from build123d import *

# Parameters (mm, degrees)
SKETCH1_W           = 75
SKETCH1_H           = 45
SKETCH1_R           = 14
SKETCH1_R_2         = 1.6
BOSS_EXTRUDE1_DEPTH = 3
FILLET2_R           = 5
SKETCH2_R           = 1.6
CUT_EXTRUDE1_DEPTH  = 44.834917589


with BuildPart() as part:
    # Sketch1 → Boss-Extrude1 (new body)
    with BuildSketch(Plane.XY):
        Rectangle(SKETCH1_W, SKETCH1_H)
        Circle(SKETCH1_R, mode=Mode.SUBTRACT)
        with Locations((-15.5, 15.5)):
            Circle(SKETCH1_R_2, mode=Mode.SUBTRACT)
        with Locations((15.5, 15.5)):
            Circle(SKETCH1_R_2, mode=Mode.SUBTRACT)
        with Locations((15.5, -15.5)):
            Circle(SKETCH1_R_2, mode=Mode.SUBTRACT)
        with Locations((-15.5, -15.5)):
            Circle(SKETCH1_R_2, mode=Mode.SUBTRACT)
    extrude(amount=BOSS_EXTRUDE1_DEPTH)

    # Fillet2
    fillet2_edges = [part.edges().sort_by_distance(p)[0] for p in [
        (37.5, -22.5, 1.5),
        (-37.5, -22.5, 1.5),
        (-37.5, 22.5, 1.5),
        (37.5, 22.5, 1.5),
    ]]
    fillet(fillet2_edges, radius=FILLET2_R)

    # Sketch2 → Cut-Extrude1 (cut, through all)
    with BuildSketch(Plane.XY.offset(3)):
        with Locations((-30, 0)):
            Circle(SKETCH2_R)
        with Locations((-30, 15)):
            Circle(SKETCH2_R)
        with Locations(Location((-30, -15, 0), (0, 0, 180))):
            Circle(SKETCH2_R)
        with Locations((30, -15)):
            Circle(SKETCH2_R)
        with Locations(Location((30, 15, 0), (0, 0, 180))):
            Circle(SKETCH2_R)
        with Locations(Location((30, 0, 0), (0, 0, 180))):
            Circle(SKETCH2_R)
    extrude(amount=-CUT_EXTRUDE1_DEPTH, mode=Mode.SUBTRACT)


solid = part.part
CAD build for the part. Positions are in the model's coordinates, mm. Round coordinates to 2 decimals unless told otherwise and drop trailing zeros. Write each loop counter-clockwise with the first axis right and the second up, starting at its lowest first coordinate (ties: lowest second). Pieces come first, ordered by that corner, then holes. Notation, with made-up numbers: (-21, 36) -> (-2, 36) arc R3 cw to (-2, 41) -> close; hole circle Ø6 at (22, -15.75). An arc over 180 degrees is marked (long way). Answer as a JSON object with one key per item and string values.
(1) Band-saw the part on D-D, the plane x = -15.5. List the corners of the cut face in (y, z).
Reported:
{"outline": "(-22.5, 0) -> (-17.1, 0) -> (-17.1, 3) -> (-22.5, 3) -> close; (-13.9, 0) -> (13.9, 0) -> (13.9, 3) -> (-13.9, 3) -> close; (17.1, 0) -> (22.5, 0) -> (22.5, 3) -> (17.1, 3) -> close"}
(2) Band-saw the part on C-C, the plane y = -8. List the corners of the cut face in (x, z).
Reported:
{"outline": "(-37.5, 0) -> (-11.49, 0) -> (-11.49, 3) -> (-37.5, 3) -> close; (11.49, 0) -> (37.5, 0) -> (37.5, 3) -> (11.49, 3) -> close"}
(3) Probe probe 1 along Y at (x, z) = (-30, 1.9); probe 2 along Y at (x, z) = (15.5, 1.4); probe 3 along X at (y, z) = (12, 2.4). List the from-to ranges inside material, lowest first. Write a range as [from, to].
Reported:
{"probe 1": "y = [-22.5, -16.6], [-13.4, -1.6], [1.6, 13.4], [16.6, 22.5]", "probe 2": "y = [-22.5, -17.1], [-13.9, 13.9], [17.1, 22.5]", "probe 3": "x = [-37.5, -7.21], [7.21, 37.5]"}
(4) Band-saw the part on B-B, the plane z = 0.85. Count the separate pieces of the cut face and the enclosed holes in it, then the cut area to 3 significant figures.
Reported:
{"separate pieces": "1", "enclosed holes": "11", "area": "2,660 mm^2"}
(5) Two-plate mould, pull along Y, no slides. Class faces 1 (the face through (-28.82, -16.08, 1.52)), 2 (the face through (-1, 15, 0)), 3 (the face through (-36.07, -21, 1.52)): +Y half, -Y half, draft (parallel to the pull), parting line (faces both ways), or undercut.
Reported:
{"face 1": "undercut", "face 2": "draft", "face 3": "-Y half"}
(6) Band-saw the part on A-A, the plane x = 30. List the corners of the cut face in (y, z).
Reported:
{"outline": "(-22.5, 0) -> (-16.6, 0) -> (-16.6, 3) -> (-22.5, 3) -> close; (-13.4, 0) -> (-1.6, 0) -> (-1.6, 3) -> (-13.4, 3) -> close; (1.6, 0) -> (13.4, 0) -> (13.4, 3) -> (1.6, 3) -> close; (16.6, 0) -> (22.5, 0) -> (22.5, 3) -> (16.6, 3) -> close"}
